```python
from build123d import *

# Parameters (mm, degrees)
M10_TAPPED_HOLE1_D     = 8.5
M10_TAPPED_HOLE1_DEPTH = 30
M10_TAPPED_HOLE1_TIP   = 2.553657631
M5_TAPPED_HOLE1_D      = 4.2
M5_TAPPED_HOLE1_DEPTH  = 20
M5_TAPPED_HOLE1_TIP    = 1.2618073


with BuildPart() as part:
    # Sketch2 → Revolve1 (revolve)
    with BuildSketch(Plane(origin=(0, 0, 0), x_dir=(1, 0, 0), z_dir=(0, 1, 0))):
        with BuildLine():
            Line((0, 70), (0, 0))
            Line((0, 0), (70, 0))
            ThreePointArc((70, 0), (49.497474683, 49.497474683), (0, 70))
        make_face()
    revolve(axis=Axis((0, 0, -70), (0, 0, 1)))

    # M10 Tapped Hole1
    with Locations(Plane.XY):
        with Locations((0, 0)):
            Hole(M10_TAPPED_HOLE1_D / 2, depth=M10_TAPPED_HOLE1_DEPTH)
            with Locations((0, 0, -(M10_TAPPED_HOLE1_DEPTH + M10_TAPPED_HOLE1_TIP / 2))):  # 118° drill point
                Cone(0, M10_TAPPED_HOLE1_D / 2, M10_TAPPED_HOLE1_TIP, mode=Mode.SUBTRACT)

    # M5 Tapped Hole1
    with Locations(Plane.XY):
        with Locations((-20, 20), (20, 20), (20, -20), (-20, -20)):
            Hole(M5_TAPPED_HOLE1_D / 2, depth=M5_TAPPED_HOLE1_DEPTH)
            with Locations((0, 0, -(M5_TAPPED_HOLE1_DEPTH + M5_TAPPED_HOLE1_TIP / 2))):  # 118° drill point
                Cone(0, M5_TAPPED_HOLE1_D / 2, M5_TAPPED_HOLE1_TIP, mode=Mode.SUBTRACT)


solid = part.part
```
Can you work these out from the model? Positions are in its coordinate system, mm. Give positions to 0.01 mm unless a question says otherwise; leave off trailing zeros. Write each loop counter-clockwise with the first axis right and the second up, starting at its lowest first coordinate (ties: lowest second). Pieces come first, ordered by that corner, then holes. Notation, with made-up numbers: (48, 79.5) - (96, 79.5) arc R20 cw to (96, 96.5) - close; hole circle Ø6 at (48.25, -32.75). An arc over 180 degrees is marked (long way). Write item = value, one per line. Start each with the question number.
1. Imagine slicing it at B-B (y = -48.5). Please give me the cut outline in (x, z).
2. Imagine slicing it at D-D (x = -27). Please give me the cut outline in (y, z).
3. Imagine slicing it at A-A (z = -10). Please give me the cut outline in (x, y).
4. For pin 1 (5 mm diameter, centred on y = 17, z = -28, fed in from -X); pin 2 (2.5 mm diameter, centred on x = -20, y = -20, fed in from -Z); pin 3 (3 mm diameter, centred on y = -30, z = -50, fed in from -X), each with a flat end and sliding along its axis, tell me the tip position at first contact or that it passes through.
5. Thinking about a two-plate mould opening in X: for faces 1 (the face through (1, -15, 0)), 2 (the face through (17.997, 20.631, -10.14)), which applies, released by +X, released by -X, zero draft, split by the parting line, or undercut?
6. Please list where these lines run through material, in increasing order: line 1 (Y direction, x = 20, z = -10); line 2 (X direction, y = 20, z = -14); line 3 (X direction, y = -20, z = -9).
7. Imagine slicing it at C-C (z = -61.5). Please give me the cut outline in (x, y), and give its area (3 significant figures).
Worked answers:
q1.outline = (-50.48, 0) arc R50.48 ccw to (50.48, 0) - close
q2.outline = (-64.58, 0) arc R64.58 ccw to (64.58, 0) - close
q3.outline = circle Ø138.56 at (0, 0); hole circle Ø4.2 at (-20, -20); hole circle Ø4.2 at (-20, 20); hole circle Ø8.5 at (0, 0); hole circle Ø4.2 at (20, -20); hole circle Ø4.2 at (20, 20)
q4.pin_1 = -63.12
q4.pin_2 = -64.57
q4.pin_3 = -40.9
q5.face_1 = zero draft
q5.face_2 = undercut
q6.line_1 = -66.33 to -22.1, -17.9 to 17.9, 22.1 to 66.33
q6.line_2 = -65.6 to -22.1, -17.9 to 17.9, 22.1 to 65.6
q6.line_3 = -66.48 to -22.1, -17.9 to 17.9, 22.1 to 66.48
q7.outline = circle Ø66.87 at (0, 0)
q7.area = 3,510 mm2
